Geometry: final body of the model. Coordinates: model frame, mm. Face numbers are marked on the shaded views. A direction names the side the tool comes from. Round coordinates to 2 decimals unless told otherwise and drop trailing zeros. Loops run counter-clockwise (first coordinate to the right, second up) from the corner with the lowest first, then second, coordinate; pieces in that order, holes last. Notation, with made-up numbers: (58, 72.5) - (86, 72.5) arc R7 ccw to (86, 81.5) - close; hole circle Ø1 at (6.25, -25). An arc over 180 degrees is marked (long way). Answer as a JSON object with one key per item and string values. Group by question number.
Item 1: Line query: line 1 (Y direction, x = 46, z = 29.5); line 2 (Y direction, x = 0, z = 2.25). Output: solid intervals per line, ascending.
Item 2: Reachability of the marked faces 5, 6 and 7 from +Z, -Z, +X, -X, +Y, -Y: full face, straight path, thin tool, end or side. Return the list, or none.
Item 3: First-contact query: pin 1 (22.5 mm diameter, centred on x = 0, y = 0, fed in from +Z); pin 2 (3 mm diameter, centred on x = -12, y = 19, fed in from +Z); pin 3 (10 mm diameter, centred on x = -54.023, y = 54.023, fed in from -Z); pin 4 (15.5 mm diameter, centred on x = 35.36, y = -35.36, fed in from +Z). Flat tips, straight axial feed; report the tip coordinate or a pass-through.
Item 4: Section B-B (x = 0). Return the cut outline in (y, z), plus the area to 3 significant figures.
Item 5: Section A-A (z = 19). Return the cut outline in (x, y), plus the area to 3 significant figures.
Item 6: Section D-D (x = 25). Return the cut outline in (y, z), plus the area to 3 significant figures.
Item 7: Draft query along X for the marked faces 1, 2, 3 and 4. Return one class per face: released by +X, released by -X, zero draft, split by the parting line, or undercut.
Autodesk Inventor part; units mm, degrees
ref_plane "YZ Plane" through (0, 0, 0) normal (1, 0, 0) x (0, 1, 0)
ref_plane "XZ Plane" through (0, 0, 0) normal (0, 1, 0) x (-1, 0, 0)
ref_plane "XY Plane" through (0, 0, 0) normal (0, 0, 1) x (1, 0, 0)
sketch "Sketch1" plane through (0, 0, 0) normal (0, 0, 1) x (1, 0, 0)
  line L0 (71, 71) -> (-71, 71)
  line L1 (-71, 71) -> (-71, -71)
  line L2 (-71, -71) -> (71, -71)
  line L3 (71, -71) -> (71, 71)
  point P0 (0, 0)
extrude "Extrusion1" add sketch "Sketch1" along normal blind 35
fillet "Fillet1" radius 5 4 edges at (-71, -71, 17.5) (-71, 71, 17.5) (71, 71, 17.5) (71, -71, 17.5)
sketch "Sketch6" plane through (0, 0, 35) normal (0, 0, 1) x (1, 0, 0)
  line L0 (-67.5, -67.5) -> (67.5, -67.5)
  line L1 (67.5, -67.5) -> (67.5, 67.5)
  line L2 (67.5, 67.5) -> (-67.5, 67.5)
  line L3 (-67.5, 67.5) -> (-67.5, -67.5)
  line L4 (-67.5, -67.5) -> (67.5, 67.5) construction
  line L5 (67.5, -67.5) -> (-67.5, 67.5) construction
  point P0 (0, 0)
  dimension "d26" = 135
  dimension "d27" = 135
extrude "Extrusion6" cut sketch "Sketch6" against normal blind 22
sketch "Sketch7" plane through (0, 0, 13) normal (0, 0, 1) x (1, 0, 0)
  point P0 (0, 0)
sketch "Sketch8" plane through (0, 0, 13) normal (0, 0, 1) x (1, 0, 0)
  circle A0 centre (0, 0) radius 55
  dimension "d30" = 110
extrude "Extrusion7" cut sketch "Sketch8" against normal blind 5
sketch "Sketch9" plane through (0, 0, 8) normal (0, 0, 1) x (1, 0, 0)
  circle A0 centre (0, 0) radius 14
  dimension "d33" = 28
extrude "Extrusion8" cut sketch "Sketch9" against normal through all
sketch "Sketch10" plane through (0, 0, 0) normal (0, 0, -1) x (-1, 0, 0)
  circle A0 centre (0, 0) radius 76.4 construction
  line L0 (0, 0) -> (54.023, -54.023) construction
  line L1 (0, 0) -> (76.4, 0) construction
  line L2 (0, 0) -> (0, -71) construction
  line L3 (66, -71) -> (-66, -71)
  line L4 (0, 0) -> (-76.4, 0) construction
  line L5 (-67.5, 67.5) -> (-67.5, -67.5)
  circle A1 centre (54.023, -54.023) radius 4.25
  circle A2 centre (-54.023, -54.023) radius 4.25
  circle A3 centre (54.023, 54.023) radius 4.25
  circle A4 centre (-54.023, 54.023) radius 4.25
  circle A5 centre (0, 0) radius 50 construction
  circle A6 centre (35.3553, -35.3553) radius 4.85
  circle A7 centre (-35.3553, -35.3553) radius 4.85
  circle A8 centre (35.3553, 35.3553) radius 4.85
  circle A9 centre (-35.3553, 35.3553) radius 4.85
  dimension "d41" = 100
  dimension "d36" = 152.8
  dimension "d37" = 45
  dimension "d38" = 8.5
  dimension "d42" = 9.7
extrude "Extrusion9" cut sketch "Sketch10" against normal through all
sketch "Sketch12" plane through (0, 0, 0) normal (0, 0, -1) x (-1, 0, 0)
  circle A0 centre (35.3553, -35.3553) radius 4.85
  circle A1 centre (35.3553, 35.3553) radius 4.85
  circle A2 centre (-35.3553, 35.3553) radius 4.85
  circle A3 centre (-35.3553, -35.3553) radius 4.85
  circle A4 centre (35.3553, -35.3553) radius 6.85
  circle A5 centre (-35.3553, -35.3553) radius 6.85
  circle A6 centre (-35.3553, 35.3553) radius 6.85
  circle A7 centre (35.3553, 35.3553) radius 6.85
  point P0 (0, 0)
extrude "Extrusion10" add sketch "Sketch12" along normal blind 5
properties part number "GEARBOX-SUPPORT" material "PET Plastic"
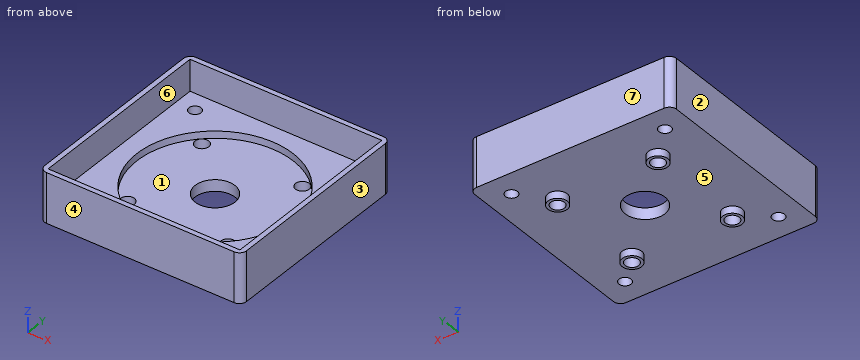
Values:
{
 "1": {"line 1": "y = -71 to -67.5, 67.5 to 71", "line 2": "y = -71 to -14, 14 to 71"},
 "2": {"face 5": "-Z", "face 6": "+Z", "face 7": "+Z, -Z, +X, -X, +Y"},
 "3": {"pin 1": "passes through", "pin 2": "stops at z = 8", "pin 3": "stops at z = 0", "pin 4": "stops at z = 13"},
 "4": {"outline": "(-71, 0) - (-14, 0) - (-14, 8) - (-55, 8) - (-55, 13) - (-67.5, 13) - (-67.5, 35) - (-71, 35) - close; (14, 0) - (71, 0) - (71, 35) - (67.5, 35) - (67.5, 13) - (55, 13) - (55, 8) - (14, 8) - close", "area": "1,230 mm^2"},
 "5": {"outline": "(-71, -66) arc R5 ccw to (-66, -71) - (66, -71) arc R5 ccw to (71, -66) - (71, 66) arc R5 ccw to (66, 71) - (-66, 71) arc R5 ccw to (-71, 66) - close; hole (-67.5, -67.5) - (67.5, -67.5) - (67.5, 67.5) - (-67.5, 67.5) - close", "area": "1,920 mm^2"},
 "6": {"outline": "(-71, 0) - (71, 0) - (71, 35) - (67.5, 35) - (67.5, 13) - (48.99, 13) - (48.99, 8) - (-48.99, 8) - (-48.99, 13) - (-67.5, 13) - (-67.5, 35) - (-71, 35) - close", "area": "1,510 mm^2"},
 "7": {"face 1": "undercut", "face 2": "released by -X", "face 3": "released by +X", "face 4": "zero draft"}
}
